Here's how the part is built. I have some questions about the finished solid (model axes, mm). Face numbers are marked on the shaded views. A direction names the side the tool comes from. Give positions to 0.01 mm unless a question says otherwise; leave off trailing zeros. Write each loop counter-clockwise with the first axis right and the second up, starting at its lowest first coordinate (ties: lowest second). Pieces come first, ordered by that corner, then holes. Notation, with made-up numbers: (-9.5, 40) -> (7.5, 40) arc R14 ccw to (7.5, 50) -> close; hole circle Ø10 at (69.25, -15). An arc over 180 degrees is marked (long way). Use CSV: the item, a comma, the result in double quotes. Start each with the question number.
(1) Suppose I cut it at A-A on y = 0. List the corners of the cut face in (x, z) for me.
(2) Suppose I cut it at B-B on z = -5. List the corners of the cut face in (x, y) for me, plus the area to 3 significant figures.
(3) For pin 1 Ø1 at (y, z) = (-14, -8) entering from +X; pin 2 Ø3 at (x, z) = (56, 7) entering from -Y; pin 3 Ø1.5 at (y, z) = (45, -7.5) entering from +X; pin 4 Ø23 at (x, y) = (0, 0) entering from -Z, each with a flat end and sliding along its axis, tell me the tip position at first contact or that it passes through.
(4) Which directions (+Z, -Z, +X, -X, +Y, -Y) give clear straight access to the entire face, cutting with the end or side of a thin tool? Please do the marked faces 5, 6 and 7.
(5) Suppose I cut it at D-D on x = -17.5. List the corners of the cut face in (y, z) for me.
(6) I need wall thicknesses on L1, parallel to X at y = -0.5, z = -6; L2, parallel to Y at x = 0, z = -0.25; L3, parallel to Y at x = 8.5, z = -6. Which ranges of each line are inside material? Lowest first, please. Write a range as [from, to].
(7) Suppose I cut it at C-C on x = -30.5. List the corners of the cut face in (y, z) for me, plus the area to 3 significant figures.
(8) If we mould it in two halves opening along Y, with no side actions, what happens to the marked faces 1, 2, 3 and 4? For each: pulls with the +Y half, pulls with the -Y half, needs draft (parallel to the pull), parting line crosses it, or undercut.
from build123d import *

# Parameters (mm, degrees)
F1_DEPTH = 15
F2_R     = 5
F3_D     = 20
F4_D     = 20


with BuildPart() as f1:
    # F0 (on Top) → F1 (new body, symmetric)
    with BuildSketch(Plane.XY):
        with BuildLine():
            Line((34.641016, 10), (-8.660254, 35))
            Line((-8.660254, 35), (3.839746, 56.650635))
            Line((3.839746, 56.650635), (-13.480762, 66.650635))
            ThreePointArc((-13.480762, 66.650635), (-38.480762, 66.650635), (-50.980762, 45))
            Line((-50.980762, 45), (-50.980762, 25))
            Line((-50.980762, 25), (-25.980762, 25))
            Line((-25.980762, 25), (-25.980762, -25))
            Line((-25.980762, -25), (-50.980762, -25))
            Line((-50.980762, -25), (-50.980762, -45))
            ThreePointArc((-50.980762, -45), (-38.480762, -66.650635), (-13.480762, -66.650635))
            Line((-13.480762, -66.650635), (3.839746, -56.650635))
            Line((3.839746, -56.650635), (-8.660254, -35))
            Line((-8.660254, -35), (34.641016, -10))
            Line((34.641016, -10), (47.141016, -31.650635))
            Line((47.141016, -31.650635), (64.461524, -21.650635))
            ThreePointArc((64.461524, -21.650635), (76.961524, 0), (64.461524, 21.650635))
            Line((64.461524, 21.650635), (47.141016, 31.650635))
            Line((47.141016, 31.650635), (34.641016, 10))
        make_face()
    extrude(amount=F1_DEPTH, both=True)

    # F2
    f2_edges = [f1.edges().sort_by_distance(p)[0] for p in [
        (12.990381, 22.5, 15),
        (12.990381, -22.5, 15),
        (-25.980762, 0, 15),
        (12.990381, 22.5, -15),
        (12.990381, -22.5, -15),
        (-25.980762, 0, -15),
        (3.839746, 56.650635, 0),
        (3.839746, -56.650635, 0),
        (47.141016, -31.650635, 0),
        (47.141016, 31.650635, 0),
        (-50.980762, -25, 0),
        (-50.980762, 25, 0),
    ]]
    fillet(f2_edges, radius=F2_R)

    # F3 (through all)
    with Locations(Plane(origin=(0, 0, 0), x_dir=(1, 0, 0), z_dir=(0, 0, -1))):
        with Locations((0, 0)):
            Hole(F3_D / 2)

    # F4 (through all)
    with Locations(Plane.XY):
        with Locations((0, 0)):
            Hole(F4_D / 2)


solid = f1.part
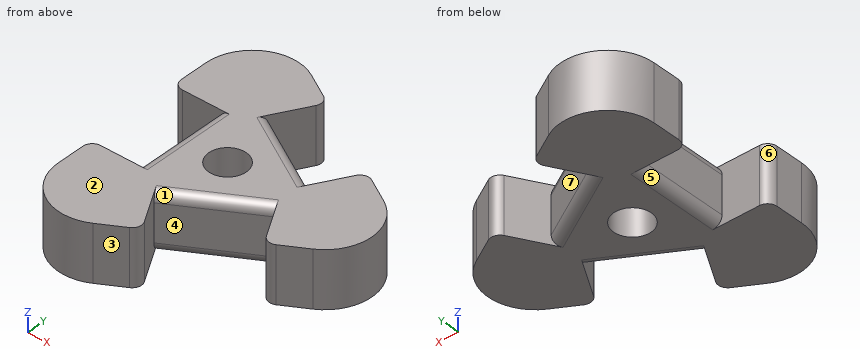
Geometry says:
1,outline,"(-25.98, -10) arc R5 ccw to (-20.98, -15) -> (-10, -15) -> (-10, 15) -> (-20.98, 15) arc R5 ccw to (-25.98, 10) -> close; (10, -15) -> (76.96, -15) -> (76.96, 15) -> (10, 15) -> close"
2,outline,"(-50.98, -45) arc R25 ccw to (-13.48, -66.65) -> (-0.49, -59.15) arc R5 ccw to (1.34, -52.32) -> (-8.66, -35) -> (34.64, -10) -> (44.64, -27.32) arc R5 ccw to (51.47, -29.15) -> (64.46, -21.65) arc R25 ccw to (64.46, 21.65) -> (51.47, 29.15) arc R5 ccw to (44.64, 27.32) -> (34.64, 10) -> (-8.66, 35) -> (1.34, 52.32) arc R5 ccw to (-0.49, 59.15) -> (-13.48, 66.65) arc R25 ccw to (-50.98, 45) -> (-50.98, 30) arc R5 ccw to (-45.98, 25) -> (-25.98, 25) -> (-25.98, -25) -> (-45.98, -25) arc R5 ccw to (-50.98, -30) -> close; hole circle Ø20 at (0, 0)"
2,area,"8,120 mm²"
3,pin 1,"x = 73"
3,pin 2,"y = -27.4"
3,pin 3,"x = -2.45"
3,pin 4,"z = -15"
4,face 5,"-Z, -X"
4,face 6,"+Z, -Z, -X"
4,face 7,"+Z, -Z"
5,outline,"(-68.52, -15) -> (68.52, -15) -> (68.52, 15) -> (-68.52, 15) -> close"
6,L1,"[-25.98, -9.99], [9.99, 76.96]"
6,L2,"[-58.83, -50], [-30, -10], [10, 30], [50, 58.83]"
6,L3,"[-25.09, -5.27], [5.27, 25.09]"
7,outline,"(-69.59, -15) -> (-25, -15) -> (-25, 15) -> (-69.59, 15) -> close; (25, -15) -> (69.59, -15) -> (69.59, 15) -> (25, 15) -> close"
7,area,"2,680 mm²"
8,face 1,"undercut"
8,face 2,"needs draft"
8,face 3,"pulls with the -Y half"
8,face 4,"undercut"
